Job drawing, mm, ordinate dimensions from the low corner. One solid piece. A direction names the side the tool comes from. Round coordinates to 2 decimals unless told otherwise and drop trailing zeros. Loops run counter-clockwise (first coordinate to the right, second up) from the corner with the lowest first, then second, coordinate; pieces in that order, holes last.
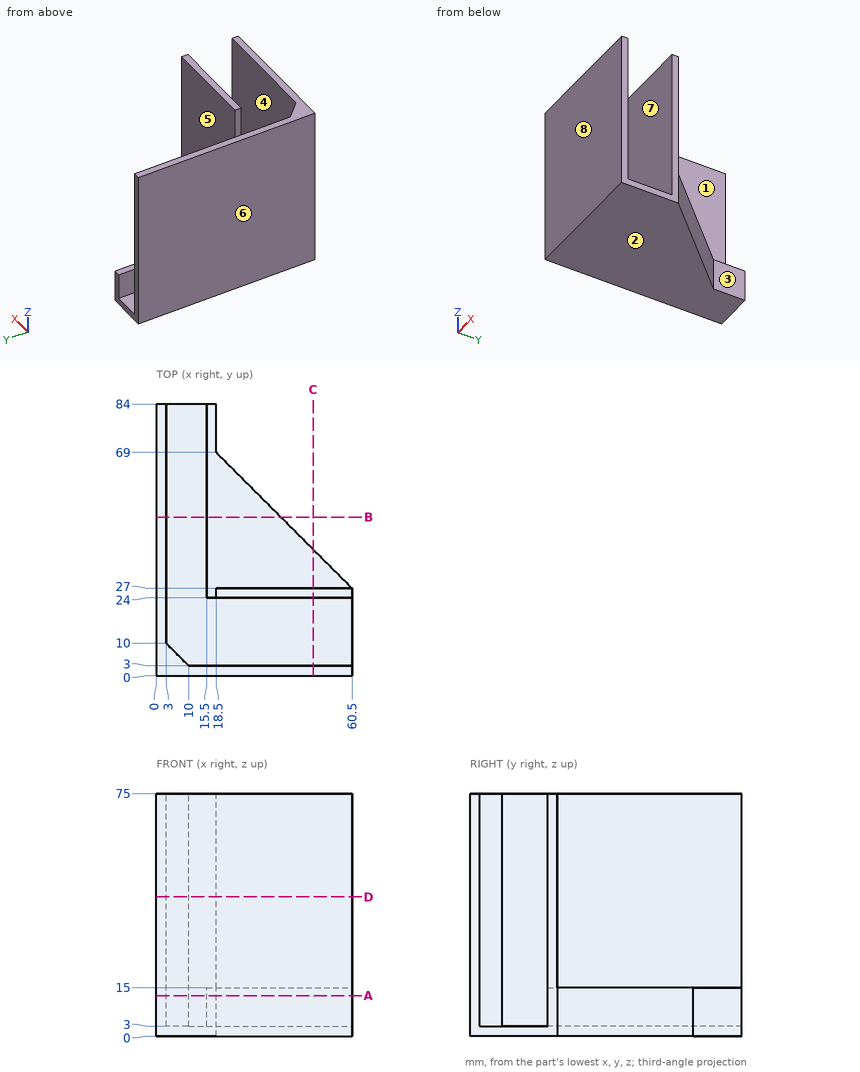
(1) Slice it at D-D on z = 43. List the corners of the cut face in (x, y).
Responses:
outline: (0, 0) - (60.5, 0) - (60.5, 3) - (10, 3) - (3, 10) - (3, 84) - (0, 84) - close; (18.5, 24) - (60.5, 24) - (60.5, 27) - (18.5, 27) - close
(2) Pin check, flat tips, straight feed: P1, Ø13.5, axis at x = 28, y = 49, coming from the +Z side; P2, Ø8, axis at x = 32, y = 8.5, coming from the +Z side; P3, Ø21.5, axis at y = 54.5, z = 52.5, coming from the +X side. Stop position of each tip, or through.
Responses:
P1: stops at z = 15
P2: stops at z = 3
P3: stops at x = 3
(3) Slice it at B-B on y = 49. List the corners of the cut face in (x, z).
Responses:
outline: (0, 0) - (38.5, 0) - (38.5, 15) - (15.5, 15) - (15.5, 3) - (3, 3) - (3, 75) - (0, 75) - close
(4) Pull direction Y, two halves, no side cores. Call the marked faces 5, 6, 7 and 8: +Y half, -Y half, draft (parallel to the pull), parting line (faces both ways), or undercut.
Responses:
face 5: +Y half
face 6: draft
face 7: undercut
face 8: -Y half
(5) Slice it at C-C on x = 48.5. List the corners of the cut face in (y, z).
Responses:
outline: (0, 0) - (39, 0) - (39, 15) - (27, 15) - (27, 75) - (24, 75) - (24, 3) - (3, 3) - (3, 75) - (0, 75) - close
(6) Which spindle directions (+Z, -Z, +X, -X, +Y, -Y) get a long thin tool onto all of the face, cutting with end or side? Do the marked faces 1, 2, 3 and 4. Say none if no direction does.
Responses:
face 1: +Z, +Y
face 2: -Z, +X, -X, +Y, -Y
face 3: +Z, -Z, +X, +Y
face 4: +Z, +X
(7) Probe line 1 (Y direction, x = 43, z = 55.5); line 2 (X direction, y = 26.5, z = 10); line 3 (X direction, y = 76, z = 60). List the from-to ranges inside material, lowest first.
Responses:
line 1: y = 0 to 3, 24 to 27
line 2: x = 0 to 3, 15.5 to 60.5
line 3: x = 0 to 3
(8) Slice it at A-A on z = 12.5. List the corners of the cut face in (x, y), plus the area to 3 significant figures.
Responses:
outline: (0, 0) - (60.5, 0) - (60.5, 3) - (10, 3) - (3, 10) - (3, 84) - (0, 84) - close; (15.5, 24) - (60.5, 24) - (60.5, 27) - (18.5, 69) - (18.5, 84) - (15.5, 84) - close
area: 1,640 mm2
